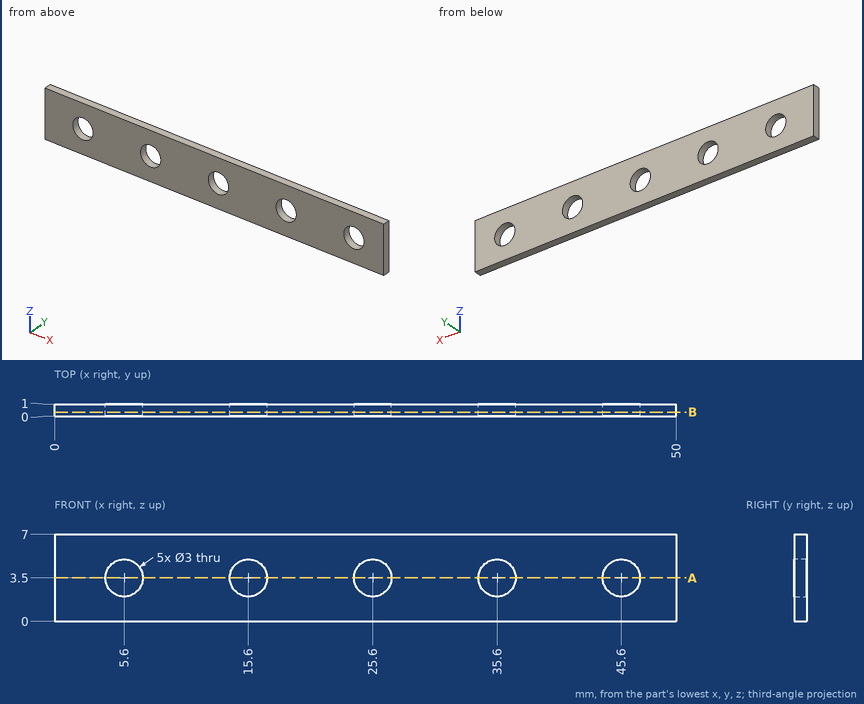
Part print with two shaded views. Sizes in mm from the minimum x, y, z corner. Coordinates: 2 decimals unless noted, no trailing zeros. Write each loop counter-clockwise with the first axis right and the second up, starting at its lowest first coordinate (ties: lowest second). Pieces come first, ordered by that corner, then holes.
(1) Cut at B-B on y = 0.35. List the corners of the cut face in (x, z), and give its area (3 significant figures).
(2) Drill centre lines: line 1 (X direction, y = 0.55, z = 3.5); line 2 (X direction, y = 0.6, z = 2.5); line 3 (Z direction, x = 24.5, y = 0.6). Where is each one in solid material? Low to high.
(3) Cut at A-A on z = 3.5. List the corners of the cut face in (x, y), and give its area (3 significant figures).
Working result:
1. outline: (0, 0) - (50, 0) - (50, 7) - (0, 7) - close; hole circle Ø3 at (5.6, 3.5); hole circle Ø3 at (15.6, 3.5); hole circle Ø3 at (25.6, 3.5); hole circle Ø3 at (35.6, 3.5); hole circle Ø3 at (45.6, 3.5)
1. area: 315 mm2
2. line 1: x = 0 to 4.1, 7.1 to 14.1, 17.1 to 24.1, 27.1 to 34.1, 37.1 to 44.1, 47.1 to 50
2. line 2: x = 0 to 4.48, 6.72 to 14.48, 16.72 to 24.48, 26.72 to 34.48, 36.72 to 44.48, 46.72 to 50
2. line 3: z = 0 to 2.48, 4.52 to 7
3. outline: (0, 0) - (4.1, 0) - (4.1, 1) - (0, 1) - close; (7.1, 0) - (14.1, 0) - (14.1, 1) - (7.1, 1) - close; (17.1, 0) - (24.1, 0) - (24.1, 1) - (17.1, 1) - close; (27.1, 0) - (34.1, 0) - (34.1, 1) - (27.1, 1) - close; (37.1, 0) - (44.1, 0) - (44.1, 1) - (37.1, 1) - close; (47.1, 0) - (50, 0) - (50, 1) - (47.1, 1) - close
3. area: 35.0 mm2
